Study the drawing (mm; zero at the part's minimum x, y, z) and answer. A direction names the side the tool comes from. Round coordinates to 2 decimals unless told otherwise and drop trailing zeros. Write each loop counter-clockwise with the first axis right and the second up, starting at its lowest first coordinate (ties: lowest second). Pieces come first, ordered by that corner, then holes.
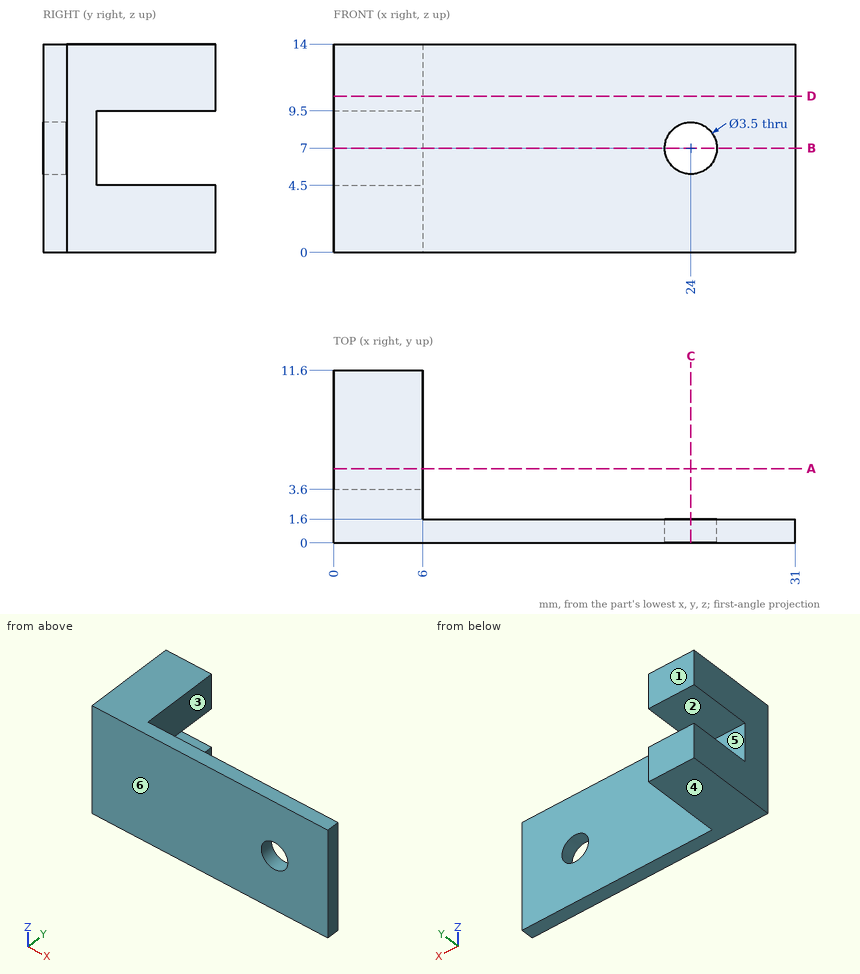
Q1. Find section B-B (z = 7). Determine the outline of the cut face in (x, y), plus the area to 3 significant figures.
Q2. Find section A-A (y = 5). Determine the outline of the cut face in (x, z), plus the area to 3 significant figures.
Q3. A tool of negligible diameter and unlimited length cuts with its end or side. For the marked faces 1, 2 and 3, from which of +Z, -Z, +X, -X, +Y, -Y can it reach the whole face along a straight path? Write none if from no direction.
Q4. Given pin 1 (1.5 mm diameter, centred on y = 7, z = 4, fed in from +X); pin 2 (2.5 mm diameter, centred on x = 4, z = 6.5, fed in from +Y), each flat-ended and moving along its own axis, determine where each tip first touches the part or whether it passes through.
Q5. Find section D-D (z = 10.5). Determine the outline of the cut face in (x, y).
Q6. Find section C-C (x = 24). Determine the outline of the cut face in (y, z), plus the area to 3 significant figures.
Q7. Find the intervals of material crossed by L1, parallel to X at y = 1.25, z = 7; L2, parallel to Z at x = 5, y = 5.25; L3, parallel to Y at x = 10.5, z = 1.5, in increasing order.
Q8. The mould has two halves that part along Z. Classify the marked faces 4, 5 and 6: +Z half, -Z half, draft (parallel to the pull), parting line (faces both ways), or undercut.
Report:
1. outline: (0, 0) - (22.25, 0) - (22.25, 1.6) - (6, 1.6) - (6, 3.6) - (0, 3.6) - close; (25.75, 0) - (31, 0) - (31, 1.6) - (25.75, 1.6) - close
1. area: 56.0 mm2
2. outline: (0, 0) - (6, 0) - (6, 4.5) - (0, 4.5) - close; (0, 9.5) - (6, 9.5) - (6, 14) - (0, 14) - close
2. area: 54.0 mm2
3. face 1: +Z, -Z, +X, -X, +Y
3. face 2: +X, -X, +Y
3. face 3: +Z, -Z, +X, +Y
4. pin 1: stops at x = 6
4. pin 2: stops at y = 3.6
5. outline: (0, 0) - (31, 0) - (31, 1.6) - (6, 1.6) - (6, 11.6) - (0, 11.6) - close
6. outline: (0, 0) - (1.6, 0) - (1.6, 5.25) - (0, 5.25) - close; (0, 8.75) - (1.6, 8.75) - (1.6, 14) - (0, 14) - close
6. area: 16.8 mm2
7. L1: x = 0 to 22.25, 25.75 to 31
7. L2: z = 0 to 4.5, 9.5 to 14
7. L3: y = 0 to 1.6
8. face 4: -Z half
8. face 5: undercut
8. face 6: draft
